from build123d import *

# Parameters (mm, degrees)
SKETCH1_W           = 800
SKETCH1_H           = 800
SKETCH1_W_2         = 760
SKETCH1_H_2         = 760
BOSS_EXTRUDE1_DEPTH = 20
SKETCH2_W           = 25.4
SKETCH2_H           = 800
BOSS_EXTRUDE2_DEPTH = 2.5
SKETCH3_W           = 2.5
SKETCH3_H           = 800
BOSS_EXTRUDE3_DEPTH = 22.9


with BuildPart() as part:
    # Sketch1 → Boss-Extrude1 (new body)
    with BuildSketch(Plane(origin=(0, 0, 0), x_dir=(1, 0, 0), z_dir=(0, 1, 0))):
        Rectangle(SKETCH1_W, SKETCH1_H)
        Rectangle(SKETCH1_W_2, SKETCH1_H_2, mode=Mode.SUBTRACT)
    extrude(amount=BOSS_EXTRUDE1_DEPTH)

    # Sketch2 → Boss-Extrude2 (add)
    with BuildSketch(Plane(origin=(0, 20, 0), x_dir=(1, 0, 0), z_dir=(0, 1, 0))):
        with Locations((83.7, 0)):
            Rectangle(SKETCH2_W, SKETCH2_H)
        with Locations((-83.7, 0)):
            Rectangle(SKETCH2_W, SKETCH2_H)
    extrude(amount=BOSS_EXTRUDE2_DEPTH)

    # Sketch3 → Boss-Extrude3 (add)
    with BuildSketch(Plane(origin=(0, 22.5, 0), x_dir=(1, 0, 0), z_dir=(0, 1, 0))):
        with Locations((-95.15, 0)):
            Rectangle(SKETCH3_W, SKETCH3_H)
        with Locations((95.15, 0)):
            Rectangle(SKETCH3_W, SKETCH3_H)
    extrude(amount=BOSS_EXTRUDE3_DEPTH)


solid = part.part
The model under review builds one solid part; all positions refer to its coordinate system, in mm. A direction names the side the tool comes from. Round coordinates to 2 decimals unless told otherwise and drop trailing zeros. Order: outer loops, then holes, each group sorted by start corner. A loop starts at its lowest first (then second) coordinate and runs counter-clockwise, first axis right, second up. Notation, with made-up numbers: (-25, -16) -> (7, -16) arc R18 cw to (7, 9) -> close; hole circle Ø10 at (4.25, 31.25). An arc over 180 degrees is marked (long way). Use CSV: the item, a comma, the result in double quotes. Start each with the question number.
(1) Tool access review of faces 1 (the face through (-93.9, 34, 6)), 2 (the face through (-384, 20, -2)), 3 (the face through (-380, 10, 5)): name each direction out of +Z, -Z, +X, -X, +Y, -Y from which nothing blocks a thin tool from reaching the whole face with its end or side.
(2) Consider section C-C on z = 92. Write out the cut boundary in (x, y), and give its area (3 significant figures).
(3) Wall thickness on probe 1 along X at (y, z) = (25, -247); probe 2 along X at (y, z) = (5, 250): over which ranges is each line inside the solid? List them lowest first. Write a range as from..to.
(4) Consider section A-A on x = 265. Write out the cut boundary in (y, z).
(5) Mouldability with a two-part tool opening along Z and no side actions: class faces 4 (the face through (-84, 20, -5)), 5 (the face through (-1, 20, -390)), 6 (the face through (-6, 12, -400)) as pulls with the +Z half, pulls with the -Z half, needs draft (parallel to the pull), parting line crosses it, or undercut.
(6) Consider section B-B on y = 37. Write out the cut boundary in (x, z).
(7) Insertion check: pin 1 (16 mm diameter, centred on x = 6.5, z = 389.5, fed in from +Y); pin 2 (11.5 mm diameter, centred on y = 29, z = -66.5, fed in from +X); pin 3 (7 mm diameter, centred on x = 82, z = -87, fed in from +Y); pin 4 (12 mm diameter, centred on y = 25.5, z = -94.5, fed in from -X). Each pin has a flat end and moves straight along its axis. Give the tip position at first contact, or say it passes through.
Responses:
1,face 1,"+Z, -Z, +Y"
1,face 2,"+Z, -Z, -X, +Y"
1,face 3,"+Y, -Y"
2,outline,"(-400, 0) -> (-380, 0) -> (-380, 20) -> (-400, 20) -> close; (-96.4, 20) -> (-71, 20) -> (-71, 22.5) -> (-93.9, 22.5) -> (-93.9, 45.4) -> (-96.4, 45.4) -> close; (71, 20) -> (96.4, 20) -> (96.4, 45.4) -> (93.9, 45.4) -> (93.9, 22.5) -> (71, 22.5) -> close; (380, 0) -> (400, 0) -> (400, 20) -> (380, 20) -> close"
2,area,"1,040 mm²"
3,probe 1,"-96.4..-93.9, 93.9..96.4"
3,probe 2,"-400..-380, 380..400"
4,outline,"(0, -400) -> (20, -400) -> (20, -380) -> (0, -380) -> close; (0, 380) -> (20, 380) -> (20, 400) -> (0, 400) -> close"
5,face 4,"undercut"
5,face 5,"needs draft"
5,face 6,"pulls with the -Z half"
6,outline,"(-96.4, -400) -> (-93.9, -400) -> (-93.9, 400) -> (-96.4, 400) -> close; (93.9, -400) -> (96.4, -400) -> (96.4, 400) -> (93.9, 400) -> close"
7,pin 1,"y = 20"
7,pin 2,"x = 96.4"
7,pin 3,"y = 22.5"
7,pin 4,"x = -400"
